Print and shaded views of the part. All mm, measured from the part's lowest x, y and z. Round coordinates to 2 decimals unless told otherwise and drop trailing zeros. Order: outer loops, then holes, each group sorted by start corner. A loop starts at its lowest first (then second) coordinate and runs counter-clockwise, first axis right, second up. Notation, with made-up numbers: M 51,62 L 74,62 A6 cw 74,71 Z; hole C 88,-35.5 d7. An arc over 180 degrees is marked long. Use CSV: the item, a comma, the result in double quotes.
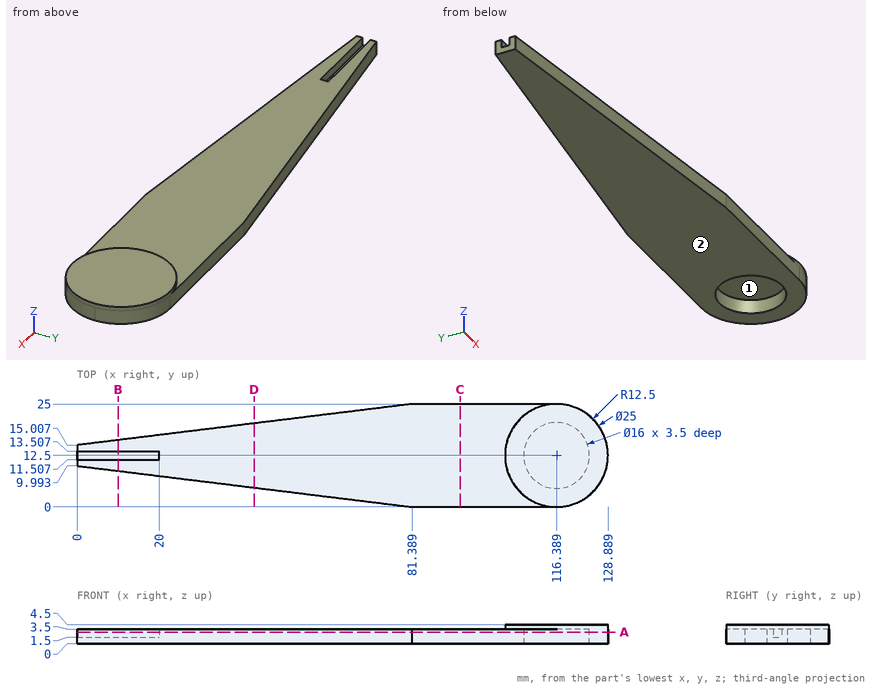
(1) Wall check: line 1 (Z direction, x = 85, y = 6.25); line 2 (Y direction, x = 109.5, z = 3.35) (1 decimal); line 3 (Y direction, x = 113.5, z = 1.1). Give the ranges that are in metal, low to high. Write a range as from..to.
Answer block:
line 1,"z = 0..3.5"
line 2,"y = 0..8.4, 16.6..25"
line 3,"y = 0..5.04, 19.96..25"
(2) Cut at A-A, the plane z = 2.8. Give the cut face in (x, y).
Answer block:
outline,"M 0,9.99 L 81.39,0 L 116.39,0 A12.5 ccw 128.89,12.5 A12.5 ccw 116.39,25 L 81.39,25 L 0,15.01 L 0,13.51 L 20,13.51 L 20,11.51 L 0,11.51 Z; hole C 116.39,12.5 d16"
(3) Cut at C-C, the plane x = 93. Give the cut face in (y, z).
Answer block:
outline,"M 0,0 L 25,0 L 25,3.5 L 0,3.5 Z"
(4) Cut at B-B, the plane x = 10. Give the cut face in (y, z) (1 decimal).
Answer block:
outline,"M 8.8,0 L 16.2,0 L 16.2,3.5 L 13.5,3.5 L 13.5,1.5 L 11.5,1.5 L 11.5,3.5 L 8.8,3.5 Z"
(5) Cut at D-D, the plane x = 43. Give the cut face in (y, z).
Answer block:
outline,"M 4.71,0 L 20.29,0 L 20.29,3.5 L 4.71,3.5 Z"
(6) Two-plate mould, pull along Y, no slides. Class the marked faces 1 and 2: released by +Y, released by -Y, zero draft, split by the parting line, or undercut.
Answer block:
face 1,"undercut"
face 2,"zero draft"
(7) Drop flat-ended pins along their axis: pin 1 (7.5 mm diameter, centred on x = 62.5, y = 18, fed in from +Z); pin 2 (2 mm diameter, centred on x = 10, z = 2, fed in from -Y); pin 3 (1 mm diameter, centred on x = 67.5, z = 2, fed in from -Y). Give the stop position or say it passes through.
Answer block:
pin 1,"stops at z = 3.5"
pin 2,"stops at y = 8.64"
pin 3,"stops at y = 1.64"
